Autodesk Inventor part; units mm, degrees
ref_plane "YZ Plane" through (0, 0, 0) normal (1, 0, 0) x (0, 1, 0)
ref_plane "XZ Plane" through (0, 0, 0) normal (0, 1, 0) x (-1, 0, 0)
ref_plane "XY Plane" through (0, 0, 0) normal (0, 0, 1) x (1, 0, 0)
sketch "Sketch1" plane through (0, 0, 0) normal (0, 0, 1) x (1, 0, 0)
  circle A0 centre (0, 0) radius 15
  dimension "d0" = 30
extrude "Extrusion1" add sketch "Sketch1" along normal blind 4
sketch "Sketch2" plane through (0, 0, 4) normal (0, 0, 1) x (1, 0, 0)
  circle A0 centre (0, 9.525) radius 1.5
  line L0 (0, -21) -> (0, 21)
  point P0 (0, 0)
  dimension "d3" = 3
  dimension "d4" = 9.525
extrude "Extrusion2" cut sketch "Sketch2" against normal blind 10
pattern_circular "Circular Pattern1" count 6 over 360 about axis through (0, 0, -10) along (0, 0, 1) of "Extrusion2"
properties part number "center_cover"
Design review of the part built by this model. Coordinates are the model's own, in mm. Give positions to 0.01 mm unless a question says otherwise; leave off trailing zeros. Loops run counter-clockwise (first coordinate to the right, second up) from the corner with the lowest first, then second, coordinate; pieces in that order, holes last. Notation, with made-up numbers: (-21, 78) -> (-7, 78) arc R30 ccw to (-7, 101) -> close; hole circle Ø8 at (17, 73). An arc over 180 degrees is marked (long way). One line per item, written item: value.
Q1. We need section B-B on y = 8.5. Give the boundary of the cut face in (x, z).
Numbers:
outline: (-12.36, 0) -> (-1.1, 0) -> (-1.1, 4) -> (-12.36, 4) -> close; (1.1, 0) -> (12.36, 0) -> (12.36, 4) -> (1.1, 4) -> close
Q2. For pin 1 Ø5 at (x, y) = (0, -9.525) entering from +Z; pin 2 Ø2 at (x, z) = (-10, 1.5) entering from +Y; pin 3 Ø2 at (x, z) = (10, 2) entering from -Y, all flat-tipped, find the tip position at first contact; note any pin that passes through.
Numbers:
pin 1: stops at z = 4
pin 2: stops at y = 12
pin 3: stops at y = -12
Q3. For L1, parallel to Y at x = 0, z = 1.6 (3 decimals); L2, parallel to Y at x = -8, z = 1.1; L3, parallel to X at y = -5.25, z = 2.1, list the stretches that pass through material, from the lowest coordinate up.
Numbers:
L1: y = -15 to -11.025, -8.025 to 8.025, 11.025 to 15
L2: y = -12.69 to -6.24, -3.28 to 3.28, 6.24 to 12.69
L3: x = -14.05 to -9.67, -6.83 to 6.83, 9.67 to 14.05
Q4. We need section C-C on z = 0.4. Give the boundary of the cut face in (x, y) (1 decimal), and give its area (3 significant figures).
Numbers:
outline: circle Ø30 at (0, 0); hole circle Ø3 at (-8.2, -4.8); hole circle Ø3 at (-8.2, 4.8); hole circle Ø3 at (0, -9.5); hole circle Ø3 at (0, 9.5); hole circle Ø3 at (8.2, -4.8); hole circle Ø3 at (8.2, 4.8)
area: 664 mm^2
Q5. We need section D-D on x = 5.5. Give the boundary of the cut face in (y, z), and give its area (3 significant figures).
Numbers:
outline: (-13.96, 0) -> (13.96, 0) -> (13.96, 4) -> (-13.96, 4) -> close
area: 112 mm^2
Q6. Draft analysis for pull direction Y (two halves, no side actions). For faces 1 (the flat face through (0, 0, 4)), 2 (the cylindrical face through (-9.354, -3.749, 2.028)), 3 (the cylindrical face through (-14.985, -0.66, 1.972)), state which applies: pulls with the +Y half, pulls with the -Y half, needs draft (parallel to the pull), parting line crosses it, or undercut.
Numbers:
face 1: needs draft
face 2: undercut
face 3: parting line crosses it
Q7. We need section A-A on x = 0. Give the boundary of the cut face in (y, z) (3 decimals).
Numbers:
outline: (-15, 0) -> (-11.025, 0) -> (-11.025, 4) -> (-15, 4) -> close; (-8.025, 0) -> (8.025, 0) -> (8.025, 4) -> (-8.025, 4) -> close; (11.025, 0) -> (15, 0) -> (15, 4) -> (11.025, 4) -> close
